Check sheet for the modelled part. Datum: model origin and axes. Units: mm. Give positions to 0.01 mm unless a question says otherwise; leave off trailing zeros. Order: outer loops, then holes, each group sorted by start corner. A loop starts at its lowest first (then second) coordinate and runs counter-clockwise, first axis right, second up.
Item 1: Release check for a two-part mould opening along X. For faces 1 (the cylindrical face through (-0.766, 9.281, 5.547)), 2 (the cylindrical face through (3.092, -5.944, 3.652)), 3 (the flat face through (5, 6, 0)), 4 (the flat face through (-12.5, 0, 4)) record: released by +X, released by -X, zero draft, split by the parting line, or undercut.
Item 2: Gauge pin test, flat ends, axial feed: P1, Ø3, axis at x = 0, z = 3.7, coming from the -Y side; P2, Ø8, axis at x = -4.5, y = -2.5, coming from the -Z side. Record the tip position at first contact, or that the pin passes through.
Item 3: Sectioned sample at C-C on x = 0. Record the boundary of the cut face in (y, z), and give its area (3 significant figures).
Item 4: Sectioned sample at A-A on z = 3.7. Record the boundary of the cut face in (x, y).
Item 5: Material ranges on line 1 along X through (y, z) = (10, 3.7); line 2 along Z through (x, y) = (0, -9.15); line 3 along Y through (x, z) = (2, 7), recorded low to high.
Item 6: Sectioned sample at B-B on y = 0. Record the boundary of the cut face in (x, z).
Item 7: Sectioned sample at D-D on y = 7.75. Record the boundary of the cut face in (x, z), and give its area (3 significant figures).
from build123d import *

# Parameters (mm, degrees)
SKETCH1_W               = 25
SKETCH1_H               = 25
SKETCH1_R               = 6.7
BOSS_EXTRUDE1_DEPTH     = 7.4
CUT_EXTRUDE1_DEPTH      = 20.164028804
CUT_EXTRUDE1_DEPTH_BACK = 20.164028804
SKETCH2_R               = 2
CHAMFER1_SIZE           = 0.25


with BuildPart() as part:
    # Sketch1 → Boss-Extrude1 (new body)
    with BuildSketch(Plane.XY):
        Rectangle(SKETCH1_W, SKETCH1_H)
        Circle(SKETCH1_R, mode=Mode.SUBTRACT)
    extrude(amount=BOSS_EXTRUDE1_DEPTH)

    # Sketch2 → Cut-Extrude1 (cut, two sides: drawn at the far end of the back side and taken through both)
    with BuildSketch(Plane(origin=(0, 0, 0), x_dir=(1, 0, 0), z_dir=(0, 1, 0)).offset(-CUT_EXTRUDE1_DEPTH_BACK)):
        with Locations(Location((0, -3.7, 0), (0, 0, 270))):
            Circle(SKETCH2_R)
    extrude(amount=CUT_EXTRUDE1_DEPTH + CUT_EXTRUDE1_DEPTH_BACK, mode=Mode.SUBTRACT)

    # Chamfer1
    chamfer1_edges = [part.edges().sort_by_distance(p)[0] for p in [
        (-6.7, 0, 0),
        (-6.7, 0, 7.4),
        (-12.5, 0, 7.4),
        (0, -12.5, 7.4),
        (0, -12.5, 1.7),
        (0, 12.5, 1.7),
        (12.5, 0, 7.4),
        (0, -12.5, 0),
        (-12.5, 0, 0),
        (0, 12.5, 0),
        (12.5, 0, 0),
        (0, 12.5, 7.4),
    ]]
    chamfer(chamfer1_edges, length=CHAMFER1_SIZE)


solid = part.part
Report:
1. face 1: undercut
1. face 2: undercut
1. face 3: zero draft
1. face 4: released by -X
2. P1: passes through
2. P2: stops at z = 0
3. outline: (-12.5, 0.25) - (-12.25, 0) - (-6.95, 0) - (-6.7, 0.25) - (-6.7, 1.7) - (-12.25, 1.7) - (-12.5, 1.45) - close; (-12.5, 5.95) - (-12.25, 5.7) - (-6.7, 5.7) - (-6.7, 7.15) - (-6.95, 7.4) - (-12.25, 7.4) - (-12.5, 7.15) - close; (6.7, 0.25) - (6.95, 0) - (12.25, 0) - (12.5, 0.25) - (12.5, 1.45) - (12.25, 1.7) - (6.7, 1.7) - close; (6.7, 5.7) - (12.25, 5.7) - (12.5, 5.95) - (12.5, 7.15) - (12.25, 7.4) - (6.95, 7.4) - (6.7, 7.15) - close
3. area: 39.1 mm2
4. outline: (-12.5, -12.5) - (-2.25, -12.5) - (-2, -12.25) - (-2, -6.39) arc R6.7 cw to (-2, 6.39) - (-2, 12.25) - (-2.25, 12.5) - (-12.5, 12.5) - close; (2, -12.25) - (2.25, -12.5) - (12.5, -12.5) - (12.5, 12.5) - (2.25, 12.5) - (2, 12.25) - (2, 6.39) arc R6.7 cw to (2, -6.39) - close
5. line 1: x = -12.5 to -2, 2 to 12.5
5. line 2: z = 0 to 1.7, 5.7 to 7.4
5. line 3: y = -12.5 to -6.39, 6.39 to 12.5
6. outline: (-12.5, 0.25) - (-12.25, 0) - (-6.95, 0) - (-6.7, 0.25) - (-6.7, 7.15) - (-6.95, 7.4) - (-12.25, 7.4) - (-12.5, 7.15) - close; (6.7, 0.25) - (6.95, 0) - (12.25, 0) - (12.5, 0.25) - (12.5, 7.15) - (12.25, 7.4) - (6.95, 7.4) - (6.7, 7.15) - close
7. outline: (-12.5, 0.25) - (-12.25, 0) - (12.25, 0) - (12.5, 0.25) - (12.5, 7.15) - (12.25, 7.4) - (-12.25, 7.4) - (-12.5, 7.15) - close; hole circle Ø4 at (0, 3.7)
7. area: 172 mm2
